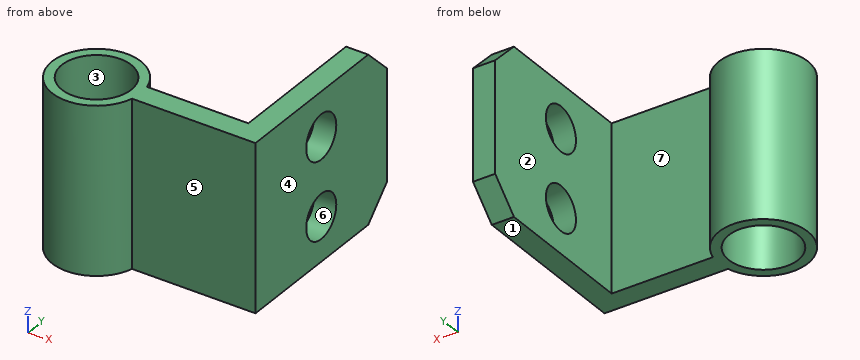
from build123d import *

# Parameters (mm, degrees)
F0_R     = 6.25
F1_DEPTH = 30
F2_R     = 4
F3_DEPTH = 38.001
F4_SIZE  = 5


with BuildPart() as f1:
    # F0 (on Top) → F1 (new body)
    with BuildSketch(Plane.XY):
        with BuildLine():
            Line((26, 2), (7.745967, 2))
            ThreePointArc((7.745967, 2), (-8, 0), (7.745967, -2))
            Line((7.745967, -2), (26, -2))
            Line((26, -2), (30, -2))
            Line((30, -2), (30, 2))
            Line((30, 2), (30, 33))
            Line((30, 33), (26, 33))
            Line((26, 33), (26, 2))
        make_face()
        Circle(F0_R, mode=Mode.SUBTRACT)
    extrude(amount=F1_DEPTH)

    # F2 (on face) → F3 (cut, through all)
    with BuildSketch(Plane.YZ.offset(30)):
        with Locations((15.5, 22)):
            Circle(F2_R)
        with Locations((15.5, 8)):
            Circle(F2_R)
    extrude(amount=-F3_DEPTH, mode=Mode.SUBTRACT)

    # F4
    f4_edges = [f1.edges().sort_by_distance(p)[0] for p in [
        (28, 33, 30),
        (28, 33, 0),
    ]]
    chamfer(f4_edges, length=F4_SIZE)


solid = f1.part
Design review of the part built by this model. Coordinates are the model's own, in mm. Face numbers are marked on the shaded views. A direction names the side the tool comes from. Coordinates: 2 decimals unless noted, no trailing zeros. Order: outer loops, then holes, each group sorted by start corner. A loop starts at its lowest first (then second) coordinate and runs counter-clockwise, first axis right, second up. Notation, with made-up numbers: (28, 31) - (66, 31) arc R20 cw to (66, 64) - close; hole circle Ø6 at (85, -38). An arc over 180 degrees is marked (long way). Put each result on its own line as item: value.
1) Take a section at D-D, the plane y = 15.5. Give the boundary of the cut face in (x, z), and give its area (3 significant figures).
Response values:
outline: (26, 0) - (30, 0) - (30, 4) - (26, 4) - close; (26, 12) - (30, 12) - (30, 18) - (26, 18) - close; (26, 26) - (30, 26) - (30, 30) - (26, 30) - close
area: 56.0 mm²
2) Take a section at A-A, the plane z = 8. Give the boundary of the cut face in (x, y), and give its area (3 significant figures).
Response values:
outline: (7.75, -2) - (30, -2) - (30, 11.5) - (26, 11.5) - (26, 2) - (7.75, 2) arc R8 ccw (long way) to start; (26, 19.5) - (30, 19.5) - (30, 33) - (26, 33) - close; hole circle Ø12.5 at (0, 0)
area: 259 mm²
3) Tool access review of the marked faces 5, 6 and 7: name each direction out of +Z, -Z, +X, -X, +Y, -Y from which nothing blocks a thin tool from reaching the whole face with its end or side.
Response values:
face 5: +Z, -Z, +X, -Y
face 6: +X, -X
face 7: +Z, -Z, +Y
4) Take a section at B-B, the plane y = 0. Give the boundary of the cut face in (x, z), and give its area (3 significant figures).
Response values:
outline: (-8, 0) - (-6.25, 0) - (-6.25, 30) - (-8, 30) - close; (6.25, 0) - (30, 0) - (30, 30) - (6.25, 30) - close
area: 765 mm²
5) Wall thickness on L1, parallel to Z at x = 27.25, y = 15.5; L2, parallel to X at y = 3, z = 11.5; L3, parallel to Y at x = 0, z = 12.25: over which ranges is each line inside the solid? List them lowest first. Write a range as from..to.
Response values:
L1: z = 0..4, 12..18, 26..30
L2: x = -7.42..-5.48, 5.48..7.42, 26..30
L3: y = -8..-6.25, 6.25..8
6) Take a section at C-C, the plane x = 0. Give the boundary of the cut face in (y, z), and give its area (3 significant figures).
Response values:
outline: (-8, 0) - (-6.25, 0) - (-6.25, 30) - (-8, 30) - close; (6.25, 0) - (8, 0) - (8, 30) - (6.25, 30) - close
area: 105 mm²
7) Insertion check: P1, Ø9, axis at y = 15.5, z = 22, coming from the -X side; P2, Ø10, axis at x = 20.5, z = 3.5, coming from the +Y side; P3, Ø1.5, axis at x = 21.5, z = 20.5, coming from the -Y side; P4, Ø3, axis at x = 18.5, y = 5, coming from the -Z side. Each pin has a flat end and moves straight along its axis. Give the tip position at first contact, or say it passes through.
Response values:
P1: stops at x = 26
P2: stops at y = 2
P3: stops at y = -2
P4: passes through
8) The part is to be moulded in two halves that separate along X. For the marked faces 1, 2, 3 and 4, say which applies: released by +X, released by -X, zero draft, split by the parting line, or undercut.
Response values:
face 1: zero draft
face 2: undercut
face 3: undercut
face 4: released by +X
